Build history of the part. All positions in model axes, mm. A direction names the side the tool comes from. Round coordinates to 2 decimals unless told otherwise and drop trailing zeros. Write each loop counter-clockwise with the first axis right and the second up, starting at its lowest first coordinate (ties: lowest second). Pieces come first, ordered by that corner, then holes.
1) Pull direction Y, two halves, no side cores. Call faces 3 (the flat face through (68, 10, -8)), 4 (the flat face through (-21, 64, 0)), 5 (the flat face through (-54.757, 53, -2)): +Y half, -Y half, draft (parallel to the pull), parting line (faces both ways), or undercut.
2) Saw through at A-A (x = -16.5). Write the cut outline in (y, z), plus the area to 3 significant figures.
3) Flat gauge pins, fed straight in: pin 1 (9 mm diameter, centred on x = -28, y = 69.5, fed in from -Z); pin 2 (5 mm diameter, centred on x = 32.5, z = -6.5, fed in from +Y); pin 3 (5 mm diameter, centred on y = 64, z = -6.5, fed in from +X). Where does each tip first touch, or does it go through?
4) Wall check: probe 1 along Y at (x, z) = (13, -12); probe 2 along Y at (x, z) = (-59.5, -2.6); probe 3 along Y at (x, z) = (60.5, -14.75). Give the ranges that are in metal, low to high.
5) Saw through at D-D (y = 42). Write the cut outline in (x, z).
6) Which spindle directions (+Z, -Z, +X, -X, +Y, -Y) get a long thin tool onto all of the face, cutting with end or side? Do faces 1 (the flat face through (-12, 54, -10)), 2 (the flat face through (42, 44.75, -13)). Say none if no direction does.
7) Saw through at B-B (y = 29). Write the cut outline in (x, z), plus the area to 3 significant figures.
Autodesk Inventor part; units mm, degrees
ref_plane "YZ Plane" through (0, 0, 0) normal (1, 0, 0) x (0, 1, 0)
ref_plane "XZ Plane" through (0, 0, 0) normal (0, 1, 0) x (-1, 0, 0)
ref_plane "XY Plane" through (0, 0, 0) normal (0, 0, 1) x (1, 0, 0)
sketch "Skizze1" plane through (0, 0, 0) normal (0, 0, 1) x (1, 0, 0)
  line L0 (-65, 0) -> (65, 0)
  line L1 (65, 0) -> (65, 20)
  line L2 (65, 20) -> (40, 20)
  line L3 (40, 20) -> (40, 54)
  line L4 (-65, 41) -> (-65, 0)
  line L5 (-65, 41) -> (-65, 41)
  line L6 (-65, 54) -> (-65, 54)
  line L7 (-65, 54) -> (-65, 41)
  line L8 (24, 71) -> (24, 54)
  line L9 (24, 54) -> (40, 54)
  circle A0 centre (-59.5, 2.832) radius 1.25
  circle A1 centre (23.1262, 2.832) radius 1.25
  circle A2 centre (23.1262, 51.168) radius 1.25
  circle A3 centre (-52.007, 51.168) radius 1.25
  line L10 (25.8762, 2.832) -> (25.8762, 0)
  line L11 (25.8762, 0) -> (20.3762, 0)
  line L12 (20.3762, 0) -> (20.3762, 2.832)
  arc A4 (25.8762, 2.832) -> (20.3762, 2.832) centre (23.1262, 2.832) ccw
  line L13 (-56.75, 0) -> (-56.75, 2.832)
  line L14 (-62.25, 0) -> (-62.25, 2.832)
  line L15 (-56.75, 0) -> (-62.25, 0)
  arc A5 (-56.75, 2.832) -> (-62.25, 2.832) centre (-59.5, 2.832) ccw
  line L16 (25.8762, 51.168) -> (25.8762, 54)
  line L17 (25.8762, 54) -> (20.3762, 54)
  line L18 (20.3762, 54) -> (20.3762, 51.168)
  arc A6 (20.3762, 51.168) -> (25.8762, 51.168) centre (23.1262, 51.168) ccw
  line L19 (-49.257, 51.168) -> (-49.257, 54)
  line L20 (-49.257, 54) -> (-54.757, 54)
  line L21 (-54.757, 54) -> (-54.757, 51.168)
  arc A7 (-54.757, 51.168) -> (-49.257, 51.168) centre (-52.007, 51.168) ccw
  line L22 (-65, 54) -> (24, 54)
  line L23 (24, 54) -> (24, 57)
  line L24 (24, 57) -> (-65, 57)
  line L25 (-65, 57) -> (-65, 54)
  line L26 (24, 71) -> (-65, 71)
  line L27 (-65, 71) -> (-65, 54)
  line L28 (43, 23) -> (68, 23)
  line L29 (68, 23) -> (68, -3)
  line L30 (68, -3) -> (-68, -3)
  line L31 (-68, -3) -> (-68, 44)
  line L32 (-68, 44) -> (-68, 44)
  line L33 (-68, 44) -> (-68, 57)
  line L34 (-68, 57) -> (-68, 57)
  line L35 (-68, 57) -> (-68, 74)
  line L36 (-68, 74) -> (27, 74)
  line L37 (27, 74) -> (27, 57)
  line L38 (27, 57) -> (43, 57)
  line L39 (43, 57) -> (43, 23)
  line L40 (-65, 71) -> (-51, 71)
  line L41 (-51, 71) -> (-51, 66)
  line L42 (-51, 66) -> (-65, 66)
  line L43 (-65, 66) -> (-65, 71)
  line L44 (8, 71) -> (-8, 71)
  line L45 (-8, 71) -> (-8, 66)
  line L46 (-8, 66) -> (8, 66)
  line L47 (8, 66) -> (8, 71)
  line L48 (-65, 71) -> (-55, 71)
  line L49 (-55, 71) -> (-55, 66)
  line L50 (-55, 66) -> (-65, 66)
  line L51 (-65, 66) -> (-65, 71)
  line L52 (1, 71) -> (-4, 71)
  line L53 (-4, 71) -> (-4, 66)
  line L54 (-4, 66) -> (1, 66)
  line L55 (1, 66) -> (1, 71)
  line L56 (8, 71) -> (1, 71)
  line L57 (1, 71) -> (1, 66)
  line L58 (1, 66) -> (8, 66)
  line L59 (8, 66) -> (8, 71)
  line L60 (-4, 71) -> (-8, 71)
  line L61 (-8, 71) -> (-8, 66)
  line L62 (-8, 66) -> (-4, 66)
  line L63 (-4, 66) -> (-4, 71)
  line L64 (8, 57) -> (-8, 57)
  line L65 (-8, 57) -> (-8, 60.5)
  line L66 (-8, 60.5) -> (8, 60.5)
  line L67 (8, 60.5) -> (8, 57)
  line L68 (1, 60.5) -> (-4, 60.5)
  line L69 (-4, 60.5) -> (-4, 57)
  line L70 (-4, 57) -> (1, 57)
  line L71 (1, 57) -> (1, 60.5)
  line L72 (-65, 57) -> (-51, 57)
  line L73 (-51, 57) -> (-51, 60.5)
  line L74 (-51, 60.5) -> (-65, 60.5)
  line L75 (-65, 60.5) -> (-65, 57)
  line L76 (-55, 60.5) -> (-65, 60.5)
  line L77 (-65, 60.5) -> (-65, 57)
  line L78 (-65, 57) -> (-55, 57)
  line L79 (-55, 57) -> (-55, 60.5)
  point P0 (0, 0)
  point P1 (0, 0)
  point P2 (0, 0)
  dimension "d0" = 130
  dimension "d1" = 25
  dimension "d8" = 20
  dimension "d9" = 41
  dimension "d11" = 54
  dimension "d42" = 5.5
  dimension "d43" = 82.6262
  dimension "d44" = 2.5
  dimension "d45" = 2.832
  dimension "d46" = 7.493
  dimension "d47" = 48.336
  dimension "d48" = 5.5
  dimension "d49" = 5.5
  dimension "d50" = 5.5
  dimension "d51" = 5.5
  dimension "d52" = 3
  dimension "d57" = 0
  dimension "d58" = 89
  dimension "d59" = 71
  dimension "d60" = 3
  dimension "d61" = 2.832
  dimension "d70" = 16
  dimension "d71" = 14
  dimension "d72" = 5
  dimension "d73" = 43
  dimension "d76" = 10
  dimension "d79" = 51
  dimension "d80" = 5
  dimension "d83" = 5.5
  dimension "d84" = 0
extrude "Extrusion1" add sketch "Skizze1" along normal blind 3 contours L4 L7 L22 L21 A7 L19 L18 A6 L16 L9 L3 L2 L1 L0 L10 A4 L12 L13 A5 L14 | L14 A5 L13 L0 | L25 L24 L8 L17 L22 L20 | L12 A4 L10 L0 | L20 L19 A7 L21 | L27 L74 L79 L24 | L79 L74 L73 L24 | L27 L42 L41 L26 L45 L46 L47 L8 L24 L67 L66 L65 L73 L74 | L17 L9 L16 A6 L18 | L27 L26 L49 L42 | L65 L66 L69 L24 | L49 L26 L41 L42 | L69 L66 L71 L24 | L24 L71 L66 L67 | L47 L46 L55 L26 | L26 L53 L46 L45 | L55 L46 L53 L26 | A0 | A1 | A2 | A3 | L28 L29 L30 L31 L33 L35 L36 L37 L38 L39
extrude "Extrusion2" add sketch "Skizze1" against normal blind 20 contours L25 L24 L8 L17 L22 L20 | L27 L26 L49 L42 | L69 L66 L71 L24 | L55 L46 L53 L26 | L28 L29 L30 L31 L33 L35 L36 L37 L38 L39
sketch "Skizze2" plane through (43, 23, 3) normal (1, 0, 0) x (0, 0, -1)
  line L0 (23, 21.75) -> (9, 21.75)
  line L1 (9, 21.75) -> (9, 9.25)
  line L2 (9, 9.25) -> (23, 9.25)
  line L3 (23, 9.25) -> (23, 21.75)
  line L4 (23, 0) -> (0, 0)
  line L5 (23, 34) -> (23, 0)
  point P0 (3, -23)
  dimension "d62" = 9.25
  dimension "d63" = 21.75
  dimension "d64" = 14
extrude "Extrusion3" cut sketch "Skizze2" against normal up to surface (3 mm away)
extrude "Extrusion6" add sketch "Skizze1" against normal blind 10 contours L27 L74 L79 L24 | L79 L74 L73 L24 | L27 L26 L49 L42 | L65 L66 L69 L24 | L49 L26 L41 L42 | L69 L66 L71 L24 | L24 L71 L66 L67 | L47 L46 L55 L26 | L26 L53 L46 L45 | L55 L46 L53 L26
extrude "Extrusion4" add sketch "Skizze1" against normal blind 4 contours L14 A5 L13 L0 | L12 A4 L10 L0 | L20 L19 A7 L21 | L17 L9 L16 A6 L18
extrude "Extrusion7" cut sketch "Skizze1" along normal blind 1.5 contours A0 | A1 | A2 | A3
sketch "Skizze3" plane through (-68, 74, 3) normal (0, 1, 0) x (1, 0, 0)
  line L0 (0, 0) -> (0, 23)
  line L1 (95, 0) -> (0, 0)
  line L2 (0, 23) -> (95, 23)
  line L3 (13, 13) -> (64, 13)
  line L4 (64, 13) -> (64, 23)
  line L5 (64, 23) -> (13, 23)
  line L6 (13, 23) -> (13, 13)
  point P0 (68, 3)
  dimension "d65" = 13
  dimension "d66" = 13
  dimension "d67" = 51
extrude "Extrusion5" cut sketch "Skizze3" against normal up to surface (3 mm away)
properties part number "Basis"
Evaluation:
1. face 3: draft
1. face 4: undercut
1. face 5: undercut
2. outline: (-3, -20) - (0, -20) - (0, 0) - (54, 0) - (54, -20) - (57, -20) - (57, 0) - (71, 0) - (71, -10) - (74, -10) - (74, 3) - (-3, 3) - close
2. area: 381 mm2
3. pin 1: stops at z = -10
3. pin 2: stops at y = 57
3. pin 3: stops at x = 27
4. probe 1: y = -3 to 0, 54 to 57, 71 to 74
4. probe 2: y = -3 to 1.58, 4.08 to 5.58, 54 to 60.5, 66 to 74
4. probe 3: y = -3 to 0, 20 to 23
5. outline: (-68, -20) - (-65, -20) - (-65, 0) - (40, 0) - (40, -6) - (43, -6) - (43, 3) - (-68, 3) - close
6. face 1: -Z
6. face 2: -Z, +X
7. outline: (-68, -20) - (-65, -20) - (-65, 0) - (40, 0) - (40, -20) - (43, -20) - (43, 3) - (-68, 3) - close
7. area: 453 mm2
